Study the drawing (mm; zero at the part's minimum x, y, z) and answer. Coordinates: 2 decimals unless noted, no trailing zeros. Write each loop counter-clockwise with the first axis right and the second up, starting at its lowest first coordinate (ties: lowest second). Pieces come first, ordered by that corner, then holes. Notation, with made-up numbers: M 80,-7 L 113,-7 A27 cw 113,17 Z; hole C 79,35.25 d5. An arc over 180 degrees is marked long. Answer as CSV lines item,"result". Start each with the question number.
(1) Find the intervals of material crossed by L1, parallel to Z at x = 31.5, y = 2.05, in increasing order. Write a range as [from, to].
(2) A cutting plane is placed at A-A on x = 38. Give the vertices of the cut face in (y, z), then the cut area to 3 significant figures.
(3) A cutting plane is placed at C-C on x = 31. Give the vertices of the cut face in (y, z), then the cut area to 3 significant figures.
(4) A cutting plane is placed at B-B on y = 2.5. Give the vertices of the cut face in (x, z).
(5) The mould has two halves that part along X. Classify the marked faces 1 and 2: released by +X, released by -X, zero draft, split by the parting line, or undercut.
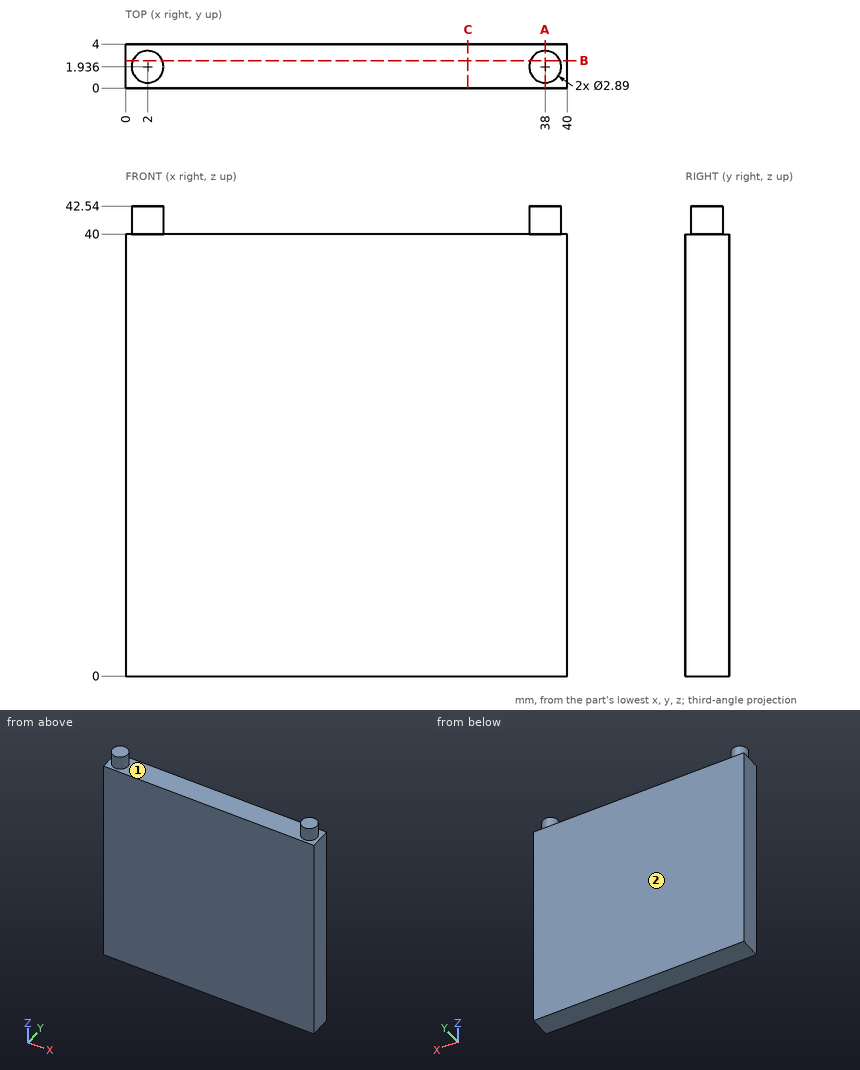
Here are the results:
1,L1,"z = [0, 40]"
2,outline,"M 0,0 L 4,0 L 4,40 L 3.38,40 L 3.38,42.54 L 0.49,42.54 L 0.49,40 L 0,40 Z"
2,area,"167 mm^2"
3,outline,"M 0,0 L 4,0 L 4,40 L 0,40 Z"
3,area,"160 mm^2"
4,outline,"M 0,0 L 40,0 L 40,40 L 39.33,40 L 39.33,42.54 L 36.67,42.54 L 36.67,40 L 3.33,40 L 3.33,42.54 L 0.67,42.54 L 0.67,40 L 0,40 Z"
5,face 1,"undercut"
5,face 2,"zero draft"
